```python
from build123d import *

# Parameters (mm, degrees)
F1_DEPTH = 25.4


with BuildPart() as f1:
    # F0 (on Front) → F1 (new body)
    with BuildSketch(Plane.XZ):
        Polygon((39.478663, 49.774494), (-42.100161, 49.774494), (-63.207971, 28.951926), (0, -40.932029), (58.875032, 30.378129), align=None)
        Polygon((-25.556205, -2.709786), (-31.747603, 7.609214), (19.511815, 2.424546), (21.704745, 0), (23.049638, -2.241488), (16.5084, -6.16623), (0, -6.16623), (-3.038761, -2.806516), (-11.864654, 0), align=None, mode=Mode.SUBTRACT)
        Polygon((0, -29.237164), (-12.149894, -17.257059), (10.827228, -18.256486), align=None, mode=Mode.SUBTRACT)
        Polygon((-52.939307, 28.666684), (-38.962513, 42.643476), (-34.113426, 42.643476), (-46.806633, 22.53401), align=None, mode=Mode.SUBTRACT)
        Polygon((40.904865, 26.38476), (40.904865, 38.364865), (50.032564, 27.810963), (38.3377, 13.26369), (30.666579, 19.430669), (19.511815, 22.676632), (7.027925, 23.939323), (-16.350178, 26.303917), (-21.210515, 26.795519), (-25.183988, 29.989879), (-25.183988, 34.941979), (-15.973477, 40.646795), (0, 42.928718), (9.698181, 40.646795), (13.976795, 36.368181), (19.226575, 26.38476), align=None, mode=Mode.SUBTRACT)
        Polygon((23.79043, 38.650107), (20.082297, 42.643476), (28.090977, 42.643476), align=None, mode=Mode.SUBTRACT)
    extrude(amount=F1_DEPTH)


solid = f1.part
```
The listing builds one solid part. Answer for the finished solid, in the listing's coordinates (mm). Round coordinates to 2 decimals unless told otherwise and drop trailing zeros. Loops run counter-clockwise (first coordinate to the right, second up) from the corner with the lowest first, then second, coordinate; pieces in that order, holes last. Notation, with made-up numbers: (8.5, 13.5) - (39.5, 13.5) arc R8 cw to (39.5, 26.5) - close; hole circle Ø6 at (-14, 24.5). An arc over 180 degrees is marked (long way). Use one line per item in the form item = value. Start each with the question number.
1. The part is cut by section D-D on z = -14. Determine the outline of the cut face in (x, y).
2. The part is cut by section A-A on z = -26.5. Determine the outline of the cut face in (x, y).
3. The part is cut by section B-B on x = 42.5. Determine the outline of the cut face in (y, z).
4. Consider line 1 (Z direction, x = -4.5, y = -12); line 2 (X direction, y = -1.5, z = 35); line 3 (X direction, y = -1.5, z = 27). Determine where each line is inside the solid, lowest interval first. Write a range as [from, to].
5. For a pull along Z with two mould halves and no side action, classify faces 1 (the face through (-52.506, -12.522, 39.509)), 2 (the face through (-32.046, -12.522, -5.501)), 3 (the face through (8, -13, -6.166)), 4 (the face through (21.96, -12.52, 40.62)) as pulls with the +Z half, pulls with the -Z half, needs draft (parallel to the pull), parting line crosses it, or undercut.
6. Given pin 1 Ø1.5 at (y, z) = (-6.5, -6.5) entering from +X; pin 2 Ø6 at (y, z) = (-3, -11) entering from -X; pin 3 Ø1.5 at (x, y) = (-35.5, -19) entering from -Z; pin 4 Ø9.5 at (y, z) = (-11, 31) entering from +X, each flat-ended and moving along its own axis, determine where each tip first touches the part or whether it passes through.
7. The part is cut by section C-C on y = -8.5. Give the number of separate pieces and of enclosed holes in the cut face, then the cut area to 3 significant figures.
Geometry check:
q1.outline = (-24.36, -25.4) - (22.24, -25.4) - (22.24, 0) - (-24.36, 0) - close
q2.outline = (-13.05, -25.4) - (-2.78, -25.4) - (-2.78, 0) - (-13.05, 0) - close; (2.7, -25.4) - (11.92, -25.4) - (11.92, 0) - (2.7, 0) - close
q3.outline = (-25.4, 10.54) - (0, 10.54) - (0, 18.44) - (-25.4, 18.44) - close; (-25.4, 36.52) - (0, 36.52) - (0, 46.75) - (-25.4, 46.75) - close
q4.line_1 = [-35.96, -24.8], [-17.59, -2.34], [4.85, 25.11], [42.29, 49.77]
q4.line_2 = [-57.08, -46.61], [-38.94, -25.09], [14.7, 40.9], [43.82, 54.25]
q4.line_3 = [-61.44, -51.27], [-43.99, -21.46], [18.9, 40.9], [49.38, 56.09]
q5.face_1 = pulls with the +Z half
q5.face_2 = pulls with the -Z half
q5.face_3 = undercut
q5.face_4 = undercut
q6.pin_1 = 29.05
q6.pin_2 = -29.79
q6.pin_3 = -2.51
q6.pin_4 = 58.88
q7.separate_pieces = 1
q7.enclosed_holes = 5
q7.area = 4,760 mm^2
